from build123d import *

# Parameters (mm, degrees)
F1_DEPTH     = 63.5
F0_W         = 25.4
F0_H         = 19.05
F2_DEPTH     = 25.4
F3_DEPTH     = 7.9375
F5_T1_DEPTH  = 50.8
F5_T3_DEPTH  = 158.75
F5_T5_DEPTH  = 53.975
F5_T7_DEPTH  = 17.4757259071
F5_T9_DEPTH  = 53.975
F5_T12_ANGLE = 147.7854112401
F5_T14_ANGLE = 147.7854112401
F5_T19_DEPTH = 53.975
F5_T23_DEPTH = 33.3507259071
F5_T30_DEPTH = 33.3507259071
F5_T34_DEPTH = 53.975


# Not quite as in the source:
# - a fillet or chamfer that OpenCascade refuses, or shapes differently, is made with other operations: its cross-section is extruded or revolved along the edge and cut away or added


with BuildPart() as f1:
    # F0 (on Front) → F1 (new body, symmetric)
    with BuildSketch(Plane.XZ):
        Polygon((-41.275, -9.525), (41.275, -9.525), (41.275, 9.525), (22.225, 9.525), (-41.275, 9.525), align=None)
    extrude(amount=F1_DEPTH, both=True)

    # F0 (on Front) → F2 (join, symmetric)
    with BuildSketch(Plane.XZ):
        with BuildLine():
            Line((22.225, 9.525), (41.275, 9.525))
            Line((41.275, 9.525), (41.275, 27.0007259071))
            ThreePointArc((41.275, 27.0007259071), (45.9704586348, 38.2716389076), (57.2792179355, 42.8752))
            Line((57.2792179355, 42.8752), (60.325, 42.8752))
            Line((60.325, 42.8752), (60.325, 61.9252))
            Line((60.325, 61.9252), (57.3416620374, 61.9252))
            add(Edge.make_bspline(
                [(53.0544398296, 61.6847569862), (54.513344238, 61.8019382233), (55.9438787453, 61.882664375), (57.3416620374, 61.9252)],
                knots=[107.5126961268, 107.5126961268, 107.5126961268, 107.5126961268, 111.6737524732, 111.6737524732, 111.6737524732, 111.6737524732], degree=3))
            ThreePointArc((53.0544398296, 61.6847569862), (31.0464268351, 50.2032924252), (22.225, 27.0007259071))
            Line((22.225, 27.0007259071), (22.225, 9.525))
        make_face()
        with Locations((73.025, 52.4002)):
            Rectangle(F0_W, F0_H)
    extrude(amount=F2_DEPTH, both=True)

    # F0 (on Front) → F3 (join, symmetric)
    with BuildSketch(Plane.XZ):
        with BuildLine():
            add(Edge.make_bspline(
                [(-41.275, 9.525), (-41.275, 31.2921475952), (15.3595053514, 58.6570472681), (53.0544398296, 61.6847569862)],
                knots=[0, 0, 0, 0, 107.5126961268, 107.5126961268, 107.5126961268, 107.5126961268], degree=3))
            Line((-41.275, 9.525), (22.225, 9.525))
            Line((22.225, 9.525), (22.225, 27.0007259071))
            ThreePointArc((22.225, 27.0007259071), (31.0464268351, 50.2032924252), (53.0544398296, 61.6847569862))
        make_face()
    extrude(amount=F3_DEPTH, both=True)

    # F0 (on Front) → F4 (revolve)
    with BuildSketch(Plane.XZ):
        Polygon((85.725, 61.9252), (85.725, 42.8752), (85.725, 38.1), (111.125, 38.1), (111.125, 66.675), (85.725, 66.675), align=None)
    revolve(axis=Axis((85.725, 0, 52.3875), (0, 0, 1)))

    # F5: fillet of radius 6.35 on 12 edges, made by hand

    # F5_s2 → F5_t1 (cut)
    with BuildSketch(Plane.XY.offset(-25.4)):
        with BuildLine():
            ThreePointArc((41.275, -57.15), (39.4151280605, -61.6401280605), (34.925, -63.5))
            Line((34.925, -63.5), (41.275, -63.5))
            Line((41.275, -63.5), (41.275, -57.15))
        make_face()
        with BuildLine():
            ThreePointArc((-34.925, -63.5), (-39.4151280605, -61.6401280605), (-41.275, -57.15))
            Line((-41.275, -57.15), (-41.275, -63.5))
            Line((-41.275, -63.5), (-34.925, -63.5))
        make_face()
        with BuildLine():
            ThreePointArc((34.925, 63.5), (39.4151280605, 61.6401280605), (41.275, 57.15))
            Line((41.275, 57.15), (41.275, 63.5))
            Line((41.275, 63.5), (34.925, 63.5))
        make_face()
        with BuildLine():
            ThreePointArc((-34.925, 63.5), (-39.4151280605, 61.6401280605), (-41.275, 57.15))
            Line((-41.275, 57.15), (-41.275, 63.5))
            Line((-41.275, 63.5), (-34.925, 63.5))
        make_face()
    extrude(amount=F5_T1_DEPTH, mode=Mode.SUBTRACT)

    # F5_s4 → F5_t3 (cut)
    with BuildSketch(Plane.XZ.offset(-79.375)):
        with BuildLine():
            ThreePointArc((34.925, -9.525), (39.4151280605, -7.6651280605), (41.275, -3.175))
            Line((41.275, -3.175), (41.275, -9.525))
            Line((41.275, -9.525), (34.925, -9.525))
        make_face()
    extrude(amount=F5_T3_DEPTH, mode=Mode.SUBTRACT)

    # F5_s6 → F5_t5 (cut)
    with BuildSketch(Plane.XZ.offset(-79.375)):
        with BuildLine():
            ThreePointArc((41.275, 3.175), (39.4151280605, 7.6651280605), (34.925, 9.525))
            Line((34.925, 9.525), (41.275, 9.525))
            Line((41.275, 9.525), (41.275, 3.175))
        make_face()
    extrude(amount=F5_T5_DEPTH, mode=Mode.SUBTRACT)

    # F5_s8 → F5_t7 (cut)
    with BuildSketch(Plane.XY.offset(9.525)):
        with BuildLine():
            ThreePointArc((41.275, 19.05), (39.4151280605, 23.5401280605), (34.925, 25.4))
            Line((34.925, 25.4), (41.275, 25.4))
            Line((41.275, 25.4), (41.275, 19.05))
        make_face()
        with BuildLine():
            ThreePointArc((41.275, -19.05), (39.4151280605, -23.5401280605), (34.925, -25.4))
            Line((34.925, -25.4), (41.275, -25.4))
            Line((41.275, -25.4), (41.275, -19.05))
        make_face()
    extrude(amount=F5_T7_DEPTH, mode=Mode.SUBTRACT)

    # F5_s10 → F5_t9 (cut)
    with BuildSketch(Plane.XZ.offset(25.4)):
        with BuildLine():
            ThreePointArc((41.275, 3.175), (39.4151280605, 7.6651280605), (34.925, 9.525))
            Line((34.925, 9.525), (41.275, 9.525))
            Line((41.275, 9.525), (41.275, 3.175))
        make_face()
    extrude(amount=F5_T9_DEPTH, mode=Mode.SUBTRACT)

    # F5_s11 → F5_t12 (revolve, cut)
    with BuildSketch(Plane.XY.offset(27.0007259071)):
        with BuildLine():
            ThreePointArc((34.925, 25.4), (39.4151280605, 23.5401280605), (41.275, 19.05))
            Line((41.275, 19.05), (41.275, 25.4))
            Line((41.275, 25.4), (34.925, 25.4))
        make_face()
    revolve(axis=Axis((57.15, 25.4, 27.0007259071), (0, 1, 0)), revolution_arc=F5_T12_ANGLE, mode=Mode.SUBTRACT)

    # F5_s13 → F5_t14 (revolve, cut)
    with BuildSketch(Plane.XY.offset(27.0007259071)):
        with BuildLine():
            ThreePointArc((41.275, -19.05), (39.4151280605, -23.5401280605), (34.925, -25.4))
            Line((34.925, -25.4), (41.275, -25.4))
            Line((41.275, -25.4), (41.275, -19.05))
        make_face()
    revolve(axis=Axis((57.15, -25.4, 27.0007259071), (0, 1, 0)), revolution_arc=F5_T14_ANGLE, mode=Mode.SUBTRACT)


with BuildPart() as f5_tool17:
    # F5_s18 → F5_t19 (new body)
    with BuildSketch(Plane.XZ.offset(-63.5)):
        with BuildLine():
            ThreePointArc((41.275, 3.175), (39.4151280605, 7.6651280605), (34.925, 9.525))
            Line((34.925, 9.525), (41.275, 9.525))
            Line((41.275, 9.525), (41.275, 3.175))
        make_face()
    extrude(amount=F5_T19_DEPTH)

    split(bisect_by=Plane.XZ.offset(-25.4), keep=Keep.TOP)


with BuildPart() as f5_tool21:
    # F5_s22 → F5_t23 (new body)
    with BuildSketch(Plane.XY.offset(-6.35)):
        with BuildLine():
            ThreePointArc((41.275, 19.05), (39.4151280605, 23.5401280605), (34.925, 25.4))
            Line((34.925, 25.4), (41.275, 25.4))
            Line((41.275, 25.4), (41.275, 19.05))
        make_face()
    extrude(amount=F5_T23_DEPTH)

    split(bisect_by=Plane.XY.offset(9.525), keep=Keep.BOTTOM)


with BuildPart() as f5_tool17_1:
    add(f5_tool17.part)

    # F5_t25: intersect F5_tool21
    add(f5_tool21.part, mode=Mode.INTERSECT)


with BuildPart() as f1_1:
    add(f1.part)

    # F5_t15: cut F5_tool17
    add(f5_tool17_1.part, mode=Mode.SUBTRACT)


with BuildPart() as f5_tool28:
    # F5_s29 → F5_t30 (new body)
    with BuildSketch(Plane.XY.offset(-6.35)):
        with BuildLine():
            ThreePointArc((41.275, -19.05), (39.4151280605, -23.5401280605), (34.925, -25.4))
            Line((34.925, -25.4), (41.275, -25.4))
            Line((41.275, -25.4), (41.275, -19.05))
        make_face()
    extrude(amount=F5_T30_DEPTH)

    split(bisect_by=Plane.XY.offset(9.525), keep=Keep.BOTTOM)


with BuildPart() as f5_tool32:
    # F5_s33 → F5_t34 (new body)
    with BuildSketch(Plane.XZ.offset(9.525)):
        with BuildLine():
            ThreePointArc((41.275, 3.175), (39.4151280605, 7.6651280605), (34.925, 9.525))
            Line((34.925, 9.525), (41.275, 9.525))
            Line((41.275, 9.525), (41.275, 3.175))
        make_face()
    extrude(amount=F5_T34_DEPTH)

    split(bisect_by=Plane.XZ.offset(25.4), keep=Keep.BOTTOM)


with BuildPart() as f5_tool28_1:
    add(f5_tool28.part)

    # F5_t36: intersect F5_tool32
    add(f5_tool32.part, mode=Mode.INTERSECT)


with BuildPart() as f1_2:
    add(f1_1.part)

    # F5_t26: cut F5_tool28
    add(f5_tool28_1.part, mode=Mode.SUBTRACT)


solid = f1_2.part
Here's how the part is built. I have some questions about the finished solid (model axes, mm). A direction names the side the tool comes from. Coordinates: 2 decimals unless noted, no trailing zeros. Loops run counter-clockwise (first coordinate to the right, second up) from the corner with the lowest first, then second, coordinate; pieces in that order, holes last.
1. Imagine slicing it at A-A, the plane z = 1. Please give me the cut outline in (x, y) (3 decimals), and give its area (3 significant figures).
2. I need wall thicknesses on L1, parallel to Y at x = -11, z = 38; L2, parallel to Y at x = 32, z = 16.5; L3, parallel to Z at x = -14, y = -25.5 (3 decimals). Which ranges of each line are inside material? Lowest first, please.
3. For faces 4 (the flat face through (46, 25.4, 48)), 5 (the flat face through (46, -25.4, 48)), 6 (the cylindrical face through (31.284, 16.547, 50.468)), 7 (the flat face through (22.225, -17, 18)), which set-ups out of +Z, -Z, +X, -X, +Y, -Y let a thin tool reach every point of the face, with its end or its side?
4. Imagine slicing it at B-B, the plane x = 95. Please give me the cut outline in (y, z) (3 decimals), and give its area (3 significant figures).
5. For P1, Ø6, axis at y = 19.5, z = 13, coming from the -X side (3 decimals); P2, Ø1.5, axis at x = -6, y = -38.5, coming from the +Z side (3 decimals); P3, Ø15.5, axis at x = 3, z = 27.5, coming from the +Y side, each with a flat end and sliding along its axis, tell me the tip position at first contact or that it passes through.
6. If we mould it in two halves opening along X, with no side actions, what happens to faces 1 (the flat face through (41.275, -1, 8)), 2 (the flat face through (60, 0, 42.875)), 3 (the flat face through (-4, 7.938, 30))? For each: pulls with the +X half, pulls with the -X half, needs draft (parallel to the pull), parting line crosses it, or undercut.
Taken from the geometry:
1. outline: (-41.275, -57.15) arc R6.35 ccw to (-34.925, -63.5) - (34.925, -63.5) arc R6.35 ccw to (41.275, -57.15) - (41.275, 57.15) arc R6.35 ccw to (34.925, 63.5) - (-34.925, 63.5) arc R6.35 ccw to (-41.275, 57.15) - close
1. area: 10,400 mm2
2. L1: y = -7.94 to 7.94
2. L2: y = -25.4 to 25.4
2. L3: z = -9.525 to 9.525
3. face 4: +Z, +X, -X, +Y
3. face 5: +Z, +X, -X, -Y
3. face 6: +Z, -X, +Y
3. face 7: +Z, -X, -Y
4. outline: (-23.646, 38.1) - (23.646, 38.1) - (23.646, 66.675) - (-23.646, 66.675) - close
4. area: 1,350 mm2
5. P1: stops at x = 22.225
5. P2: stops at z = 9.525
5. P3: stops at y = 7.94
6. face 1: pulls with the +X half
6. face 2: undercut
6. face 3: needs draft
